from build123d import *

# Parameters (mm, degrees)
F0_W      = 127
F0_H      = 127
F1_DEPTH  = 25.4
F2_T      = -6.35
F3_SIZE   = 7.62
F5_DEPTH  = 127.001
F6_W      = 10
F6_H      = 12
F7_DEPTH  = 0.3175
F8_W      = 10
F8_H      = 12
F9_DEPTH  = 0.3175
F11_DEPTH = 127.001


with BuildPart() as f1:
    # F0 (on Top) → F1 (new body)
    with BuildSketch(Plane.XY):
        Rectangle(F0_W, F0_H)
    extrude(amount=F1_DEPTH)

    # F2
    f2_openings = [f1.faces().sort_by_distance(p)[0] for p in [
        (0, 0, 25.4),
    ]]
    offset(amount=F2_T, openings=f2_openings)

    # F3
    f3_edges = [f1.edges().sort_by_distance(p)[0] for p in [
        (-63.5, -63.5, 12.7),
        (63.5, -63.5, 12.7),
        (63.5, 63.5, 12.7),
        (-63.5, 63.5, 12.7),
        (-57.15, 57.15, 15.875),
        (57.15, 57.15, 15.875),
        (57.15, -57.15, 15.875),
        (-57.15, -57.15, 15.875),
    ]]
    chamfer(f3_edges, length=F3_SIZE)

    # F4 (on face) → F5 (cut, through all)
    with BuildSketch(Plane(origin=(-63.5, 0, 0), x_dir=(0, -1, 0), z_dir=(-1, 0, 0))):
        with BuildLine():
            ThreePointArc((42.4942, 8.753), (41.8692, 8.128), (42.4942, 7.503))
            Line((42.4942, 7.503), (42.4942, 8.753))
        make_face()
        with BuildLine():
            ThreePointArc((42.4942, 17.897), (41.8692, 17.272), (42.4942, 16.647))
            Line((42.4942, 16.647), (42.4942, 17.897))
        make_face()
        with BuildLine():
            Line((42.4942, 17.897), (42.4942, 16.647))
            ThreePointArc((42.4942, 16.647), (42.9361417382, 16.8300582618), (43.1192, 17.272))
            ThreePointArc((43.1192, 17.272), (42.9361417382, 17.7139417382), (42.4942, 17.897))
        make_face()
        with BuildLine():
            ThreePointArc((42.4942, 14.45), (40.7442, 12.7), (42.4942, 10.95))
            Line((42.4942, 10.95), (42.4942, 12.7))
            Line((42.4942, 12.7), (42.4942, 14.45))
        make_face()
        with BuildLine():
            Line((42.4942, 12.7), (42.4942, 10.95))
            ThreePointArc((42.4942, 10.95), (43.7316368671, 11.4625631329), (44.2442, 12.7))
            Line((44.2442, 12.7), (42.4942, 12.7))
        make_face()
        with BuildLine():
            Line((42.4942, 8.753), (42.4942, 7.503))
            ThreePointArc((42.4942, 7.503), (42.9361417382, 7.6860582618), (43.1192, 8.128))
            ThreePointArc((43.1192, 8.128), (42.9361417382, 8.5699417382), (42.4942, 8.753))
        make_face()
        with BuildLine():
            Line((42.4942, 14.45), (42.4942, 12.7))
            Line((42.4942, 12.7), (44.2442, 12.7))
            ThreePointArc((44.2442, 12.7), (43.7316368671, 13.9374368671), (42.4942, 14.45))
        make_face()
    extrude(amount=-F5_DEPTH, mode=Mode.SUBTRACT)

    # F6 (on face) → F7 (cut)
    with BuildSketch(Plane.YZ.offset(-57.15)):
        with Locations((-42.4942, 12.7)):
            Rectangle(F6_W, F6_H)
    extrude(amount=-F7_DEPTH, mode=Mode.SUBTRACT)

    # F8 (on face) → F9 (cut)
    with BuildSketch(Plane(origin=(57.15, 0, 0), x_dir=(0, -1, 0), z_dir=(-1, 0, 0))):
        with Locations((42.4942, 12.7)):
            Rectangle(F8_W, F8_H)
    extrude(amount=-F9_DEPTH, mode=Mode.SUBTRACT)

    # F10 (on face) → F11 (cut, through all)
    with BuildSketch(Plane(origin=(-63.5, 0, 0), x_dir=(0, -1, 0), z_dir=(-1, 0, 0))):
        with BuildLine():
            ThreePointArc((-42.4942, 14.45), (-44.2442, 12.7), (-42.4942, 10.95))
            Line((-42.4942, 10.95), (-42.4942, 14.45))
        make_face()
        with BuildLine():
            Line((-42.4942, 14.45), (-42.4942, 10.95))
            ThreePointArc((-42.4942, 10.95), (-41.2567631329, 11.4625631329), (-40.7442, 12.7))
            ThreePointArc((-40.7442, 12.7), (-41.2567631329, 13.9374368671), (-42.4942, 14.45))
        make_face()
    extrude(amount=-F11_DEPTH, mode=Mode.SUBTRACT)


solid = f1.part
Design review of the part built by this model. Coordinates are the model's own, in mm. A direction names the side the tool comes from. Give positions to 0.01 mm unless a question says otherwise; leave off trailing zeros. Loops run counter-clockwise (first coordinate to the right, second up) from the corner with the lowest first, then second, coordinate; pieces in that order, holes last. Notation, with made-up numbers: (22.25, 70) - (58.25, 70) arc R19 cw to (58.25, 88) - close; hole circle Ø9 at (89, 8). An arc over 180 degrees is marked (long way). Write item = value, one per line.
1) Tool access review of faces 4 (the face through (57.468, -41, 14)), 5 (the face through (57.15, -1, 16)), 6 (the face through (59.64, 59.74, 12.52)): name each direction out of +Z, -Z, +X, -X, +Y, -Y from which nothing blocks a thin tool from reaching the whole face with its end or side.
Result sheet:
face_4 = none
face_5 = +Z
face_6 = +Z, -Z, +X, +Y
2) To check wall thickness, follow line 1 (Y direction, x = -29, z = 24.25); line 2 (X direction, y = -38, z = 12.5). State the ranges of each line that lie inside material, in increasing order.
Result sheet:
line_1 = -63.5 to -57.15, 57.15 to 63.5
line_2 = -63.5 to -57.47, 57.47 to 63.5
3) Draft analysis for pull direction Y (two halves, no side actions). For faces 1 (the face through (-1, 1, 0)), 2 (the face through (-1, -57.15, 16)), 3 (the face through (59.74, -59.64, 12.52)), state which applies: +Y half, -Y half, draft (parallel to the pull), parting line (faces both ways), or undercut.
Result sheet:
face_1 = draft
face_2 = undercut
face_3 = -Y half
4) Clearance check with a flat-ended pin moving along its axis: pin 1 Ø5 at (x, y) = (49, -1.5) entering from +Z. State where the tip first meets the part, or that it passes through.
Result sheet:
pin_1 = 6.35
5) Take a section at B-B on y = 12. State the section outline as (x, z) points.
Result sheet:
outline = (-63.5, 0) - (63.5, 0) - (63.5, 25.4) - (57.15, 25.4) - (57.15, 6.35) - (-57.15, 6.35) - (-57.15, 25.4) - (-63.5, 25.4) - close
6) Take a section at A-A on z = 20.5. State the section outline as (x, y) points.
Result sheet:
outline = (-63.5, -55.88) - (-55.88, -63.5) - (55.88, -63.5) - (63.5, -55.88) - (63.5, 55.88) - (55.88, 63.5) - (-55.88, 63.5) - (-63.5, 55.88) - close; hole (-57.15, -49.53) - (-49.53, -57.15) - (49.53, -57.15) - (57.15, -49.53) - (57.15, 49.53) - (49.53, 57.15) - (-49.53, 57.15) - (-57.15, 49.53) - close
